Verification items for the finished model (mm, model axes). Face numbers are marked on the shaded views. Coordinates: 2 decimals unless noted, no trailing zeros. Order: outer loops, then holes, each group sorted by start corner. A loop starts at its lowest first (then second) coordinate and runs counter-clockwise, first axis right, second up. Notation, with made-up numbers: M -19.75,-9 L 28.25,-9 A21 cw 28.25,17 Z; hole C 59.5,52.5 d5. An arc over 180 degrees is marked long. Write item = value, one per line.
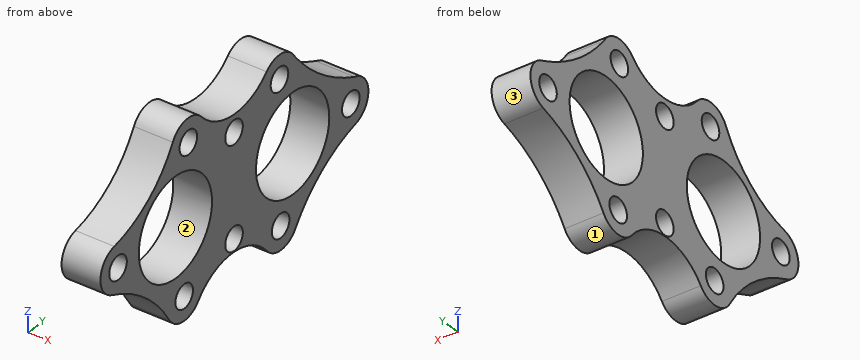
Autodesk Inventor part; units mm, degrees
ref_plane "YZ Plane" through (0, 0, 0) normal (1, 0, 0) x (0, 1, 0)
ref_plane "XZ Plane" through (0, 0, 0) normal (0, 1, 0) x (-1, 0, 0)
ref_plane "XY Plane" through (0, 0, 0) normal (0, 0, 1) x (1, 0, 0)
sketch "Sketch2" plane through (0, 0, 0) normal (1, 0, 0) x (0, 1, 0)
  circle A0 centre (0, 0) radius 12.5
  line L0 (0, 0) -> (40, 0)
  circle A1 centre (40, 0) radius 12.5
  arc A2 (61.4867, -6.219) -> (61.2036, 5.4037) centre (59.8596, -0.4438) ccw
  circle A3 centre (59.8596, -0.4438) radius 3
  arc A4 (8.9245, 22.4355) -> (-0.904, 21.2616) centre (4.4125, 18.4805) ccw
  arc A5 (-2.1636, -21.4445) -> (7.7329, -22.0405) centre (2.9878, -18.3684) ccw
  arc A6 (31.2492, -21.7764) -> (40.9283, -21.2885) centre (35.9106, -17.9987) ccw
  arc A7 (40.7702, 20.8389) -> (36.9681, 12.1267) centre (35.5128, 17.9476) ccw
  line L1 (20, 0) -> (20, -13)
  line L2 (20, 0) -> (20, 13)
  arc A8 (-18.8462, 6.1399) -> (-21.6016, -5.4642) centre (-19.5799, 0.1849) ccw
  circle A9 centre (4.4125, 18.4805) radius 3
  circle A10 centre (2.9878, -18.3684) radius 3
  circle A11 centre (35.9106, -17.9987) radius 3
  circle A12 centre (35.5128, 17.9476) radius 3
  circle A13 centre (-19.5799, 0.1849) radius 3
  circle A14 centre (20, -13) radius 3
  circle A15 centre (20, 13) radius 3
  arc A16 (8.9245, 22.4355) -> (31.139, 22.0548) centre (20.2045, 32.323) ccw
  arc A17 (31.2492, -21.7764) -> (7.7329, -22.0405) centre (19.5956, -31.2207) ccw
  arc A18 (-2.1636, -21.4445) -> (-21.6016, -5.4642) centre (-34.1581, -40.5495) ccw
  arc A19 (-20.855, 6.0479) -> (-0.904, 21.2616) centre (-27.1495, 34.9909) ccw
  arc A20 (61.4867, -6.219) -> (40.9283, -21.2885) centre (71.3527, -41.2366) ccw
  arc A21 (7.2664, 17.5556) -> (-1.5702, 18.935) centre (0, 0) ccw
  arc A22 (40.7702, 20.8389) -> (61.2036, 5.4037) centre (79.072, 50.3008) ccw
  point P0 (-18.7745, -6.6085)
  point P1 (-17.6848, 6.9242)
  dimension "d4" = 25
  dimension "d22" = 6
  dimension "d1" = 25
  dimension "d3" = 40
  dimension "d6" = 12
  dimension "d7" = 6
  dimension "d12" = 12
  dimension "d13" = 12
  dimension "d15" = 12
  dimension "d16" = 12
  dimension "d17" = 13
  dimension "d18" = 13
  dimension "d21" = 12
  dimension "d23" = 6
  dimension "d24" = 6
  dimension "d25" = 6
  dimension "d26" = 6
  dimension "d27" = 6
  dimension "d28" = 6
  dimension "d29" = 15
  dimension "d30" = 15
  dimension "d31" = 37.2645
  dimension "d34" = 36.3809
extrude "Extrusion1" add sketch "Sketch2" along normal mid plane 10
properties part number "hw6"
Item 1: Sectioned sample at B-B, the plane x = 0. Give the number of separate pieces and of enclosed holes in the cut face, then the cut area to 3 significant figures.
Report:
separate_pieces = 1
enclosed_holes = 10
area = 1,560 mm^2
Item 2: Scan lines: L1, parallel to Z at x = 0.75, y = 20; L2, parallel to Y at x = 4, z = 17; L3, parallel to Z at x = 0.25, y = 7. Record each from-to range of solid material in increasing order. Write a range as from..to.
Report:
L1 = -16.23..-16, -10..10, 16..17.32
L2 = -3.62..1.8, 7.02..32.67, 38.36..44.06
L3 = -22.83..-10.36, 10.36..16.96, 20..23.89
Item 3: Sectioned sample at A-A, the plane y = 20. Enter the section's corners in (x, z).
Report:
outline = M -5,-16.23 L 5,-16.23 L 5,-16 L -5,-16 Z; M -5,-10 L 5,-10 L 5,10 L -5,10 Z; M -5,16 L 5,16 L 5,17.32 L -5,17.32 Z
Item 4: Gauge pin test, flat ends, axial feed: pin 1 (4 mm diameter, centred on x = -1, z = 11.5, fed in from -Y); pin 2 (6 mm diameter, centred on x = -1.5, y = 22.5, fed in from +Z); pin 3 (1.5 mm diameter, centred on x = -1.5, z = 2.5, fed in from -Y). Record the tip position at first contact, or that the pin passes through.
Report:
pin_1 = -12.07
pin_2 = 18.29
pin_3 = -25.37
Item 5: Release check for a two-part mould opening along Z. For the marked faces 1, 2 and 3 record: pulls with the +Z half, pulls with the -Z half, needs draft (parallel to the pull), parting line crosses it, or undercut.
Report:
face_1 = pulls with the -Z half
face_2 = undercut
face_3 = parting line crosses it
